Read the model definition and answer for the solid it produces. Units are mm, in the model's axes. Give positions to 0.01 mm unless a question says otherwise; leave off trailing zeros. Write each loop counter-clockwise with the first axis right and the second up, starting at its lowest first coordinate (ties: lowest second). Pieces come first, ordered by that corner, then holes.
```python
from build123d import *

# Parameters (mm, degrees)
SKETCH1_W           = 198.582793441
SKETCH1_H           = 434.599999988
BOSS_EXTRUDE1_DEPTH = 12.7
CUT_EXTRUDE1_REACH  = 14.7
SKETCH2_W           = 141.287862113
SKETCH2_H           = 32.775
CUT_EXTRUDE2_REACH  = 14.7
HOLE1_D             = 3.175
HOLE1_DEPTH         = 38.1
HOLE1_CSINK_D       = 10.16
HOLE1_CSINK_ANGLE   = 82
HOLE1_TIP           = 0.953866233


with BuildPart() as part:
    # Sketch1 → Boss-Extrude1 (new body)
    with BuildSketch(Plane.XY):
        with Locations((17.439596016, 0)):
            Rectangle(SKETCH1_W, SKETCH1_H)
    extrude(amount=BOSS_EXTRUDE1_DEPTH)

    # Sketch2 → Cut-Extrude1 (cut, up to next)
    with BuildSketch(Plane(origin=(0, 0, 0), x_dir=(-1, 0, 0), z_dir=(0, 0, -1)), mode=Mode.PRIVATE) as cut_extrude1_sk1:
        with Locations((11.207869649, 200.912499994)):
            Rectangle(SKETCH2_W, SKETCH2_H)
    cut_extrude1_tool1 = extrude(cut_extrude1_sk1.sketch, amount=-CUT_EXTRUDE1_REACH, mode=Mode.PRIVATE) & part.part
    add(cut_extrude1_tool1.solids().sort_by_distance((-11.20787, 200.9125, 0))[0], mode=Mode.SUBTRACT)
    # Sketch2 → Cut-Extrude1 (cut, up to next)
    with BuildSketch(Plane(origin=(0, 0, 0), x_dir=(-1, 0, 0), z_dir=(0, 0, -1)), mode=Mode.PRIVATE) as cut_extrude1_sk2:
        with Locations((11.207869649, -200.912499994)):
            Rectangle(SKETCH2_W, SKETCH2_H)
    cut_extrude1_tool2 = extrude(cut_extrude1_sk2.sketch, amount=-CUT_EXTRUDE1_REACH, mode=Mode.PRIVATE) & part.part
    add(cut_extrude1_tool2.solids().sort_by_distance((-11.20787, -200.9125, 0))[0], mode=Mode.SUBTRACT)

    # Sketch3 → Cut-Extrude2 (cut, up to next)
    with BuildSketch(Plane.XY.offset(12.7), mode=Mode.PRIVATE) as cut_extrude2_sk1:
        Polygon((62.611061408, 94.249999997), (-56.451800705, 94.249999997), (-56.451800705, 184.524999994), (-81.851800705, 184.524999994), (-81.851800705, 94.249999997), (-85.026800705, 94.249999997), (-85.026800705, -94.249999997), (-81.851800705, -94.249999997), (-81.851800705, -184.524999994), (-56.451800705, -184.524999994), (-56.451800705, -94.249999997), (62.611061408, -94.249999997), align=None)
    cut_extrude2_tool1 = extrude(cut_extrude2_sk1.sketch, amount=-CUT_EXTRUDE2_REACH, mode=Mode.PRIVATE) & part.part
    add(cut_extrude2_tool1.solids().sort_by_distance((-19.405412, 0, 12.7))[0], mode=Mode.SUBTRACT)

    # Hole1
    with Locations(Plane(origin=(449.828463103, 0, 12.7), x_dir=(0, 1, 0), z_dir=(0, 0, 1))):
        with Locations((-108.649999997, 355.39493603), (108.649999997, 355.39493603), (207.774999994, 355.39493603), (174.999999994, 448.336332751), (135.266666663, 384.042401694), (176.283333328, 384.042401694), (-174.999999994, 448.336332751), (-135.266666663, 384.042401694), (-176.283333328, 384.042401694), (-207.774999994, 355.39493603)):
            CounterSinkHole(HOLE1_D / 2, HOLE1_CSINK_D / 2, depth=HOLE1_DEPTH, counter_sink_angle=HOLE1_CSINK_ANGLE)
            with Locations((0, 0, -(HOLE1_DEPTH + HOLE1_TIP / 2))):  # 118° drill point
                Cone(0, HOLE1_D / 2, HOLE1_TIP, mode=Mode.SUBTRACT)


solid = part.part
```
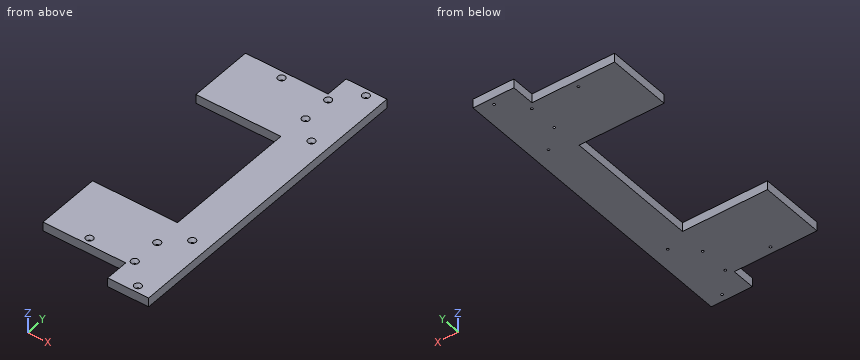
Item 1: Section C-C (y = 15) is taken. Write down the section's boundary in (x, z).
Result set:
outline: (62.61, 0) - (116.73, 0) - (116.73, 12.7) - (62.61, 12.7) - close
Item 2: Find the intervals of material crossed by line 1 along Y through (x, z) = (-34, 3) (3 decimals); line 2 along Y through (x, z) = (0.5, 10) (3 decimals); line 3 along X through (y, z) = (175, 3), in increasing order.
Result set:
line 1: y = -184.525 to -94.25, 94.25 to 184.525
line 2: y = -184.525 to -177.546, -172.454 to -94.25, 94.25 to 172.454, 177.546 to 184.525
line 3: x = -56.45 to -0.1, 3.08 to 64.85, 66.72 to 116.73
Item 3: Section B-B (z = 10.75) is taken. Give the number of separate pieces and of enclosed holes in the cut face, and give its area (3 significant figures).
Result set:
separate pieces: 1
enclosed holes: 10
area: 44,900 mm2
Item 4: Each of these flat-tipped pins is pushed along its axis until it touches: pin 1 Ø5 at (x, y) = (94.43, 108.65) entering from +Z; pin 2 Ø3 at (x, y) = (65.79, 176.28) entering from +Z; pin 3 Ø4 at (y, z) = (10, 5) entering from -X; pin 4 Ø4 at (x, y) = (65.79, -176.28) entering from +Z. Where does it stop, or does it pass through?
Result set:
pin 1: stops at z = 9.74
pin 2: passes through
pin 3: stops at x = 62.61
pin 4: stops at z = 9.16
Item 5: Section A-A (x = 45) is taken. Write down the section's boundary in (y, z) (3 decimals).
Result set:
outline: (-184.525, 0) - (-94.25, 0) - (-94.25, 12.7) - (-184.525, 12.7) - close; (94.25, 0) - (184.525, 0) - (184.525, 12.7) - (94.25, 12.7) - close
